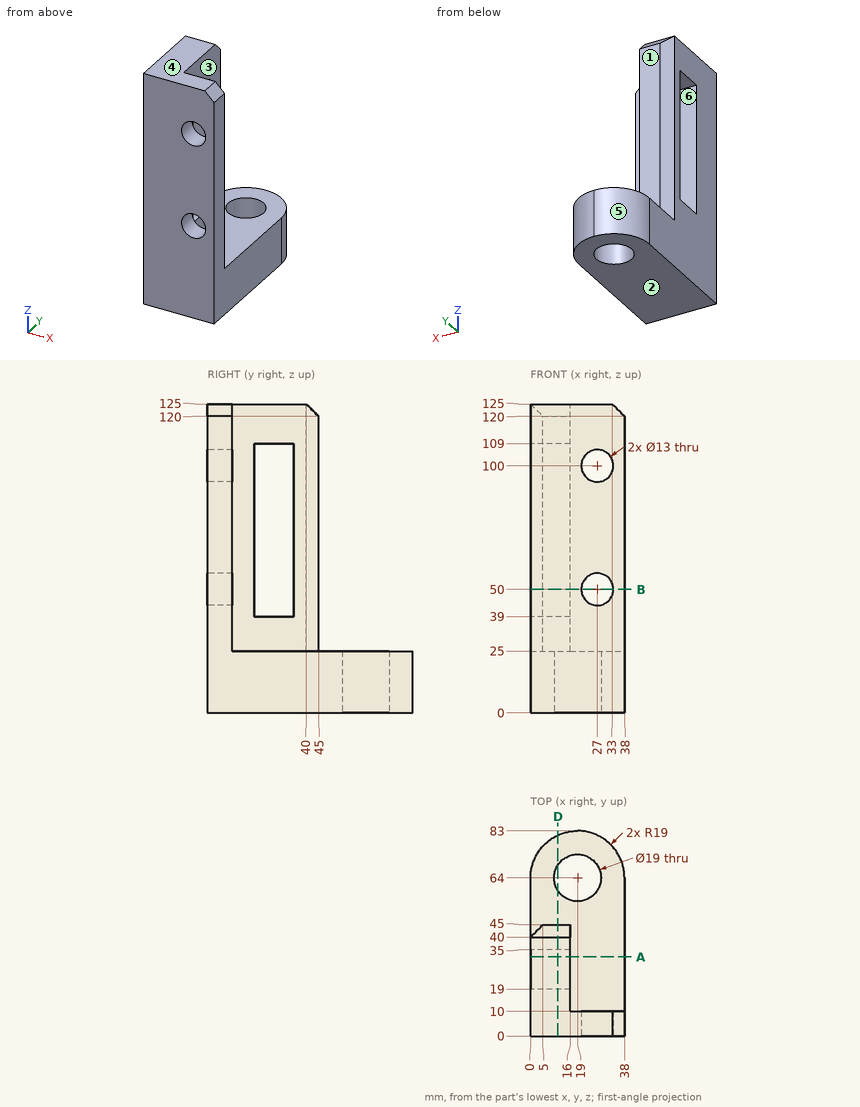
Here's the drawing with two shaded views (mm, measured from the low corner). I have some questions. A direction names the side the tool comes from. Coordinates: 2 decimals unless noted, no trailing zeros. Write each loop counter-clockwise with the first axis right and the second up, starting at its lowest first coordinate (ties: lowest second). Pieces come first, ordered by that corner, then holes. Notation, with made-up numbers: M 76,-19 L 100,-19 A30 ccw 100,16 Z; hole C 51.5,79 d9. An arc over 180 degrees is marked long. Use one line per item in the form item = value.
Q1. For the marked faces 1, 2 and 3, which set-ups out of +Z, -Z, +X, -X, +Y, -Y let a thin tool reach every point of the face, with its end or its side?
Model answer:
face_1 = +Z, +X, -X, +Y
face_2 = -Z, +X, -X, +Y, -Y
face_3 = +Z, +X, +Y
Q2. We'd pull the mould along Y, two halves only. Please class the marked faces 4, 5 and 6: +Y half, -Y half, draft (parallel to the pull), parting line (faces both ways), or undercut.
Model answer:
face_4 = draft
face_5 = +Y half
face_6 = undercut
Q3. I need wall thicknesses on line 1 along Z through (x, y) = (27, 5.5); line 2 along Y through (x, z) = (15, 94); line 3 along Z through (x, y) = (9.5, 34). Which ranges of each line are inside material? Lowest first, please. Write a range as from..to.
Model answer:
line_1 = 0..43.5, 56.5..93.5, 106.5..125
line_2 = 0..19, 35..45
line_3 = 0..39, 109..125
Q4. For P1, Ø6.5, axis at x = 26, z = 70.5, coming from the +Y side; P2, Ø10, axis at x = 28, y = 54.5, coming from the +Z side; P3, Ø11.5, axis at x = 21, y = 46, coming from the +Z side, each with a flat end and sliding along its axis, tell me the tip position at first contact or that it passes through.
Model answer:
P1 = 10
P2 = 25
P3 = 121.84
Q5. If we section it at A-A (y = 32): Write out the boundary of the cut face in (x, z).
Model answer:
outline = M 0,0 L 38,0 L 38,25 L 16,25 L 16,39 L 0,39 Z; M 0,109 L 16,109 L 16,125 L 0,125 Z
Q6. If we section it at D-D (x = 11): Write out the boundary of the cut face in (y, z), then the cut area to 3 significant figures.
Model answer:
outline = M 0,0 L 58.88,0 L 58.88,25 L 45,25 L 45,120 L 40,125 L 0,125 Z; M 69.12,0 L 81.23,0 L 81.23,25 L 69.12,25 Z; hole M 19,39 L 35,39 L 35,109 L 19,109 Z
area = 5,140 mm^2
Q7. If we section it at B-B (z = 50): Write out the boundary of the cut face in (x, y).
Model answer:
outline = M 0,0 L 20.5,0 L 20.5,10 L 16,10 L 16,19 L 0,19 Z; M 0,35 L 16,35 L 16,45 L 5,45 L 0,40 Z; M 33.5,0 L 38,0 L 38,10 L 33.5,10 Z
